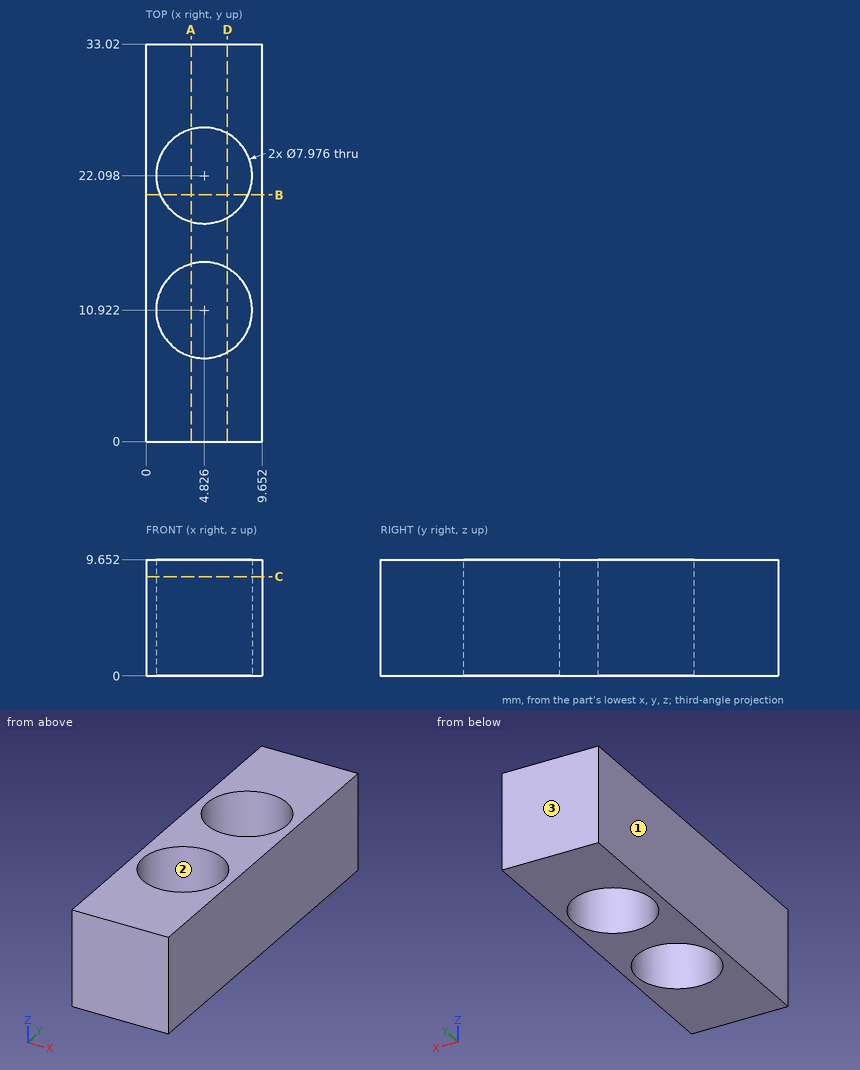
Could you check a few things on this drawing? It's one solid part, dimensions in mm from its lowest x, y, z. Round coordinates to 2 decimals unless told otherwise and drop trailing zeros. Order: outer loops, then holes, each group sorted by start corner. A loop starts at its lowest first (then second) coordinate and runs counter-clockwise, first axis right, second up. Notation, with made-up numbers: M -4,36 L 3,36 A31 cw 3,73 Z; hole C 34.5,-16 d1. An arc over 180 degrees is marked long. Return JSON: item names as keys, results as strings. Group by question number.
1. If we section it at A-A on x = 3.75: List the corners of the cut face in (y, z) for me.
2. If we section it at D-D on x = 6.75: List the corners of the cut face in (y, z) for me (1 decimal).
3. I'm going to push flat-ended pins straight in: pin 1 Ø2 at (x, z) = (5, 6.5) entering from -Y; pin 2 Ø5 at (x, y) = (5.5, 10) entering from -Z. Where does each tip first touch, or does it pass through?
4. If we section it at C-C on z = 8.25: List the corners of the cut face in (x, y) for me (1 decimal).
5. If we section it at B-B on y = 20.5: List the corners of the cut face in (x, z) for me.
6. If we mould it in two halves opening along X, with no side actions, what happens to the marked faces 1, 2 and 3? For each: pulls with the +X half, pulls with the -X half, needs draft (parallel to the pull), parting line crosses it, or undercut.
7. Please list where these lines run through material, in increasing order: probe 1 along Y at (x, z) = (3, 6.25); probe 2 along Y at (x, z) = (4, 8.25); probe 3 along X at (y, z) = (12, 1) (1 decimal).
Reply:
{
 "1": {"outline": "M 0,0 L 7.08,0 L 7.08,9.65 L 0,9.65 Z; M 14.76,0 L 18.26,0 L 18.26,9.65 L 14.76,9.65 Z; M 25.94,0 L 33.02,0 L 33.02,9.65 L 25.94,9.65 Z"},
 "2": {"outline": "M 0,0 L 7.4,0 L 7.4,9.7 L 0,9.7 Z; M 14.4,0 L 18.6,0 L 18.6,9.7 L 14.4,9.7 Z; M 25.6,0 L 33,0 L 33,9.7 L 25.6,9.7 Z"},
 "3": {"pin 1": "y = 0", "pin 2": "through"},
 "4": {"outline": "M 0,0 L 9.7,0 L 9.7,33 L 0,33 Z; hole C 4.8,10.9 d8; hole C 4.8,22.1 d8"},
 "5": {"outline": "M 0,0 L 1.17,0 L 1.17,9.65 L 0,9.65 Z; M 8.48,0 L 9.65,0 L 9.65,9.65 L 8.48,9.65 Z"},
 "6": {"face 1": "pulls with the -X half", "face 2": "undercut", "face 3": "needs draft"},
 "7": {"probe 1": "0 to 7.38, 14.47 to 18.55, 25.64 to 33.02", "probe 2": "0 to 7.02, 14.82 to 18.2, 26 to 33.02", "probe 3": "0 to 1, 8.7 to 9.7"}
}
